from build123d import *

# Parameters (mm, degrees)
ESBO_O1_W                = 387.6
ESBO_O1_H                = 320
RESSALTO_EXTRUS_O1_DEPTH = 6
CORTE_EXTRUS_O1_DEPTH    = 503.662670187
ESBO_O3_R                = 14.25
CORTE_EXTRUS_O2_DEPTH    = 503.662670187
FILETE1_R                = 144
FILETE2_R                = 144
ESBO_O4_W                = 6
ESBO_O4_H                = 50
RESSALTO_EXTRUS_O2_DEPTH = 31.4
ESBO_O5_W                = 25.4
ESBO_O5_H                = 50
CORTE_EXTRUS_O3_DEPTH    = 528.25420828
ESBO_O6_W                = 40
ESBO_O6_H                = 80
CORTE_EXTRUS_O4_DEPTH    = 528.25420828
FILETE3_R                = 5
CHANFRO1_SIZE            = 1
FILETE4_R                = 1
ESBO_O8_R                = 3
CORTE_EXTRUS_O5_DEPTH    = 527.945845339


with BuildPart() as part:
    # Esboço1 → Ressalto-extrusão1 (new body)
    with BuildSketch(Plane.XY):
        with Locations((193.8, 160)):
            Rectangle(ESBO_O1_W, ESBO_O1_H)
    extrude(amount=RESSALTO_EXTRUS_O1_DEPTH)

    # Esboço2 → Corte-extrusão1 (cut, through all)
    with BuildSketch(Plane.XY.offset(6)):
        Polygon((33.8, 320), (103.8, 200), (283.8, 200), (353.8, 320), align=None)
    extrude(amount=-CORTE_EXTRUS_O1_DEPTH, mode=Mode.SUBTRACT)

    # Esboço3 → Corte-extrusão2 (cut, through all)
    with BuildSketch(Plane.XY.offset(6)):
        with Locations((43.8, 234)):
            Circle(ESBO_O3_R)
        with Locations(Location((343.8, 234, 0), (0, 0, 180))):
            Circle(ESBO_O3_R)
    extrude(amount=-CORTE_EXTRUS_O2_DEPTH, mode=Mode.SUBTRACT)

    # Filete1
    # the kernel refuses this fillet: 144 mm, written as the material it takes off along each edge
    with BuildSketch(Plane(origin=(353.8, 320, 180.735732562), x_dir=(1, 0, 0), z_dir=(0, 0, -1))) as filete1_piece_1:
        with BuildLine():
            CenterArc((89.166452625, 132.930643283), FILETE1_R, 210.256437164, 37.131526626)
            Line((-35.217709105, 60.373215608), (-37.705392339, 58.922067054))
            Line((-37.705392339, 58.922067054), (-2.487683235, -1.451148554))
            Line((-2.487683235, -1.451148554), (0, -2.88))
            ThreePointArc((0, -2.88), (16.9, -2.88), (32.692670948, -2.658612866))
            Line((32.692670948, -2.658612866), (33.8, 0))
        make_face()
    extrude(amount=355.471465124, mode=Mode.SUBTRACT)
    with BuildSketch(Plane(origin=(33.8, 320, 180.735732562), x_dir=(-1, 0, 0), z_dir=(0, 0, -1))) as filete1_piece_2:
        with BuildLine():
            CenterArc((89.166452625, -132.930643283), FILETE1_R, 112.612036211, 37.131526626)
            Line((-35.217709105, -60.373215608), (-37.705392339, -58.922067054))
            Line((-37.705392339, -58.922067054), (-2.487683235, 1.451148554))
            Line((-2.487683235, 1.451148554), (0, 2.88))
            ThreePointArc((0, 2.88), (16.9, 2.88), (32.692670948, 2.658612866))
            Line((32.692670948, 2.658612866), (33.8, 0))
        make_face()
    extrude(amount=355.471465124, mode=Mode.SUBTRACT)

    # Filete2
    filete2_edges = [part.edges().sort_by_distance(p)[0] for p in [
        (283.8, 200, 3),
        (103.8, 200, 3),
    ]]
    fillet(filete2_edges, radius=FILETE2_R)

    # Esboço4 → Ressalto-extrusão2 (add)
    with BuildSketch(Plane.ZY):
        with Locations((3, 236.902997942)):
            Rectangle(ESBO_O4_W, ESBO_O4_H)
        with Locations((3, 136.902997942)):
            Rectangle(ESBO_O4_W, ESBO_O4_H)
        with Locations((3, 36.902997942)):
            Rectangle(ESBO_O4_W, ESBO_O4_H)
    ressalto_extrus_o2 = extrude(amount=RESSALTO_EXTRUS_O2_DEPTH)

    # Espelhar1: Ressalto-extrusão2 across plane
    add(ressalto_extrus_o2.mirror(Plane.ZY.offset(-193.8)))

    # Esboço5 → Corte-extrusão3 (cut, through all)
    with BuildSketch(Plane.XY.offset(6)):
        with Locations((406.3, 36.902997942)):
            Rectangle(ESBO_O5_W, ESBO_O5_H)
        with Locations((-18.7, 136.902997942)):
            Rectangle(ESBO_O5_W, ESBO_O5_H)
    extrude(amount=-CORTE_EXTRUS_O3_DEPTH, mode=Mode.SUBTRACT)

    # Esboço6 → Corte-extrusão4 (cut, through all)
    with BuildSketch(Plane.XY.offset(6)):
        with Locations((373.6, 40)):
            Rectangle(ESBO_O6_W, ESBO_O6_H)
    extrude(amount=-CORTE_EXTRUS_O4_DEPTH, mode=Mode.SUBTRACT)

    # Filete3
    filete3_edges = [part.edges().sort_by_distance(p)[0] for p in [
        (387.6, 80, 3),
        (353.6, 80, 3),
        (353.6, 0, 3),
    ]]
    fillet(filete3_edges, radius=FILETE3_R)

    # Chanfro1
    chanfro1_edges = [part.edges().sort_by_distance(p)[0] for p in [
        (-31.4, 61.902997942, 3),
        (-31.4, 11.902997942, 3),
        (419, 261.902997942, 3),
        (419, 211.902997942, 3),
        (419, 161.902997942, 3),
        (419, 111.902997942, 3),
        (-31.4, 261.902997942, 3),
        (-31.4, 211.902997942, 3),
    ]]
    chamfer(chanfro1_edges, length=CHANFRO1_SIZE)

    # Filete4
    filete4_edges = [part.edges().sort_by_distance(p)[0] for p in [
        (0, 320, 3),
        (387.6, 320, 3),
    ]]
    fillet(filete4_edges, radius=FILETE4_R)

    # Esboço8 → Corte-extrusão5 (cut, through all)
    with BuildSketch(Plane.XY.offset(6)):
        with Locations((407.9, 253.902997942)):
            Circle(ESBO_O8_R)
        with Locations((407.9, 219.902997942)):
            Circle(ESBO_O8_R)
        with Locations((407.9, 153.902997942)):
            Circle(ESBO_O8_R)
        with Locations((407.9, 119.902997942)):
            Circle(ESBO_O8_R)
        with Locations((-20.3, 19.902997942)):
            Circle(ESBO_O8_R)
        with Locations((-20.3, 53.902997942)):
            Circle(ESBO_O8_R)
        with Locations((-20.3, 219.902997942)):
            Circle(ESBO_O8_R)
        with Locations((-20.3, 253.902997942)):
            Circle(ESBO_O8_R)
    extrude(amount=-CORTE_EXTRUS_O5_DEPTH, mode=Mode.SUBTRACT)


solid = part.part
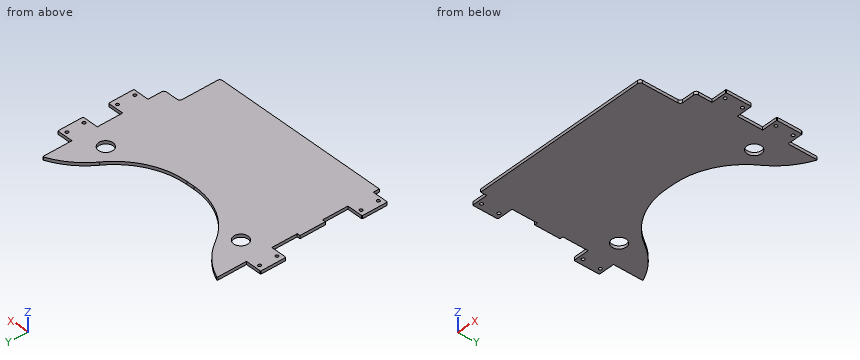
Model file for the job. Use its own axes, mm. Round coordinates to 2 decimals unless told otherwise and drop trailing zeros. Loops run counter-clockwise (first coordinate to the right, second up) from the corner with the lowest first, then second, coordinate; pieces in that order, holes last. Notation, with made-up numbers: M -29,-23 L -22,-23 A35 cw -22,16 Z; hole C 48.25,-20.5 d5. An arc over 180 degrees is marked long. One line per question, with ' | ' between items.
1) Band-saw the part on C-C (y = 234). Give the number of separate pieces and of enclosed holes in the cut face, then the cut area to 3 significant figures.
Solved:
separate pieces: 4 | enclosed holes: 0 | area: 1,150 mm²
2) Flat gauge pins, fed straight in: pin 1 (1.8 mm diameter, centred on y = 198, z = 3.5, fed in from -X); pin 2 (3.5 mm diameter, centred on x = 407.9, y = 153.9, fed in from +Z); pin 3 (1.8 mm diameter, centred on x = 400.5, z = 4, fed in from -Y). Where does each tip first touch, or does it go through?
Solved:
pin 1: stops at x = 0 | pin 2: passes through | pin 3: stops at y = 111.9
3) Band-saw the part on B-B (y = 295). Give the cut face in (x, z).
Solved:
outline: M 0,0 L 39.96,0 L 39.96,6 L 0,6 Z; M 347.64,0 L 387.6,0 L 387.6,6 L 347.64,6 Z
4) Drill centre lines: line 1 along Y through (x, z) = (407.9, 3.45); line 2 along X through (y, z) = (236, 0.75); line 3 along X through (y, z) = (35.5, 2.25). Where is each one in solid material? Low to high.
Solved:
line 1: y = 111.9 to 116.9, 122.9 to 150.9, 156.9 to 161.9, 211.9 to 216.9, 222.9 to 250.9, 256.9 to 261.9 | line 2: x = -31.4 to 29.69, 57.91 to 90.88, 296.72 to 329.69, 357.91 to 419 | line 3: x = -31.4 to 353.6
5) Band-saw the part on A-A (x = 343.8). Give the cut face in (y, z), then the cut area to 3 significant figures.
Solved:
outline: M 0,0 L 219.75,0 L 219.75,6 L 0,6 Z; M 248.25,0 L 291.48,0 L 291.48,6 L 248.25,6 Z | area: 1,580 mm²
